from build123d import *

# Parameters (mm, degrees)
SKETCH1_R           = 4
BOSS_EXTRUDE1_DEPTH = 30
SKETCH8_R           = 4
SKETCH8_R_2         = 3
CUT_EXTRUDE2_DEPTH  = 25
SKETCH15_R          = 3
SKETCH15_R_2        = 2.5
CUT_EXTRUDE3_DEPTH  = 15
THREAD1_PITCH       = 1
SKETCH18_R          = 2.5
BOSS_EXTRUDE2_DEPTH = 4


with BuildPart() as part:
    # Sketch1 → Boss-Extrude1 (new body)
    with BuildSketch(Plane(origin=(0, 0, 0), x_dir=(1, 0, 0), z_dir=(0, 1, 0))):
        with Locations(Location((0, 0, 0), (0, 0, 270))):
            Circle(SKETCH1_R)
    extrude(amount=BOSS_EXTRUDE1_DEPTH)

    # Sketch8 → Cut-Extrude2 (cut)
    with BuildSketch(Plane.XZ):
        with Locations(Location((0, 0, 0), (0, 0, 270))):
            Circle(SKETCH8_R)
        with Locations(Location((0, 0, 0), (0, 0, 270))):
            Circle(SKETCH8_R_2, mode=Mode.SUBTRACT)
    extrude(amount=-CUT_EXTRUDE2_DEPTH, mode=Mode.SUBTRACT)

    # Sketch15 → Cut-Extrude3 (cut)
    with BuildSketch(Plane.XZ):
        with Locations(Location((0, 0, 0), (0, 0, 270))):
            Circle(SKETCH15_R)
        with Locations(Location((0, 0, 0), (0, 0, 270))):
            Circle(SKETCH15_R_2, mode=Mode.SUBTRACT)
    extrude(amount=-CUT_EXTRUDE3_DEPTH, mode=Mode.SUBTRACT)

    # Thread1: the profile of Thread Profile1 profile screwed along a right-hand helix of 6 turns, 8 arcs to a turn; built about Z, then put on its axis
    thread1_z = Axis((0, 0, 0), (0, 0, 1))
    thread1_corners = [(3.0003, 0, -0.000173205), (3.0003, 0, 0.875173202), (2.458734125, 0, 0.562499999), (2.458734125, 0, 0.312499999)]
    with BuildLine(mode=Mode.PRIVATE) as thread1_profile:
        Line(thread1_corners[0], thread1_corners[1])
        Line(thread1_corners[1], thread1_corners[2])
        Line(thread1_corners[2], thread1_corners[3])
        Line(thread1_corners[3], thread1_corners[0])
    thread1_cap = Face(thread1_profile.wire())
    thread1_turn_angles = [0, 22.5, 45, 67.5, 90, 112.5, 135, 157.5, 180, 202.5, 225, 247.5, 270, 292.5, 315, 337.5, 360]
    thread1_turn_weights = [1, 0.9238795325112867, 1, 0.9238795325112867, 1, 0.9238795325112867, 1, 0.9238795325112867, 1, 0.9238795325112867, 1, 0.9238795325112867, 1, 0.9238795325112867, 1, 0.9238795325112867, 1]
    thread1_turn_rails = [Edge.make_bspline([Vector(p[0], p[1], 0).rotate(thread1_z, thread1_turn_angles[k]) / thread1_turn_weights[k] + Vector(0, 0, p[2] + THREAD1_PITCH * thread1_turn_angles[k] / 360) for k in range(17)], [0, 0, 0, 1, 1, 2, 2, 3, 3, 4, 4, 5, 5, 6, 6, 7, 7, 8, 8, 8], 2, thread1_turn_weights) for p in thread1_corners]
    thread1_turn_sides = [Face.make_surface_from_curves(thread1_turn_rails[p[0]], thread1_turn_rails[p[1]]) for p in [(0, 1), (1, 2), (2, 3), (3, 0)]]
    thread1_turn = Solid(Shell([*thread1_turn_sides, thread1_cap, thread1_cap.rotate(thread1_z, 360).moved(Location((0, 0, THREAD1_PITCH * 360 / 360)))]))
    thread1_each = [*[thread1_turn.moved(Location((0, 0, THREAD1_PITCH * i))) for i in range(6)]]
    add(Plane(origin=(0, 15, 0), x_dir=(1, 0, 0), z_dir=(0, 1, 0)) * Compound([thread1_each[i] for i in range(0, 6, 2)]), mode=Mode.SUBTRACT)
    add(Plane(origin=(0, 15, 0), x_dir=(1, 0, 0), z_dir=(0, 1, 0)) * Compound([thread1_each[i] for i in range(1, 6, 2)]), mode=Mode.SUBTRACT)

    # Sketch18 → Boss-Extrude2 (add)
    with BuildSketch(Plane(origin=(0, 30, 0), x_dir=(1, 0, 0), z_dir=(0, 1, 0))):
        with Locations(Location((0, 0, 0), (0, 0, 90))):
            Circle(SKETCH18_R)
    extrude(amount=BOSS_EXTRUDE2_DEPTH)


solid = part.part
CAD build for the part. Positions are in the model's coordinates, mm. A direction names the side the tool comes from. Coordinates: 2 decimals unless noted, no trailing zeros. Write each loop counter-clockwise with the first axis right and the second up, starting at its lowest first coordinate (ties: lowest second). Pieces come first, ordered by that corner, then holes. Notation, with made-up numbers: (4, -31) - (34, -31) arc R29 ccw to (34, -2) - close; hole circle Ø10 at (28.25, 10). An arc over 180 degrees is marked (long way). Use a Markdown table: item, result. Add a question column.
Item 1: Flat gauge pins, fed straight in: pin 1 (2 mm diameter, centred on y = 22.5, z = 0.5, fed in from -X); pin 2 (3 mm diameter, centred on y = 10.5, z = 0, fed in from -X). Where does each tip first touch, or does it go through?
Item 2: Drill centre lines: L1, parallel to Y at x = -2.25, z = 2.25; L2, parallel to X at y = 10.5, z = 0; L3, parallel to X at y = 14.5, z = -1.25. Where is each one in solid material? Low to high. Write a range as from..to.
Item 3: Band-saw the part on B-B, the plane y = 29. Give the cut face in (x, z), and give its area (3 significant figures).
Item 4: Band-saw the part on A-A, the plane y = 32.5. Give the cut face in (x, z), and give its area (3 significant figures).
Item 5: 3-axis set-ups, long thin cutter, end or side, ignore diameter. For faces 1 (the face through (-3.905, 27.465, -0.867)), 2 (the face through (-2.44, 7.4, 0.54)), 3 (the face through (2, 30, 2)): which of +Z, -Z, +X, -X, +Y, -Y reach the whole face in a straight line?
Numbers:
| question | item | result |
|---|---|---|
| 1 | pin 1 | x = -3 |
| 1 | pin 2 | x = -2.5 |
| 2 | L1 | 25..30 |
| 2 | L2 | -2.5..2.5 |
| 2 | L3 | -2.17..2.17 |
| 3 | outline | circle Ø8 at (0, 0) |
| 3 | area | 50.3 mm2 |
| 4 | outline | circle Ø5 at (0, 0) |
| 4 | area | 19.6 mm2 |
| 5 | face 1 | +Y, -Y |
| 5 | face 2 | -Y |
| 5 | face 3 | +Y |
